Autodesk Inventor part; units mm, degrees
ref_plane "YZ Plane" through (0, 0, 0) normal (1, 0, 0) x (0, 1, 0)
ref_plane "XZ Plane" through (0, 0, 0) normal (0, 1, 0) x (-1, 0, 0)
ref_plane "XY Plane" through (0, 0, 0) normal (0, 0, 1) x (1, 0, 0)
sketch "Sketch1" plane through (0, 0, 0) normal (0, 0, 1) x (1, 0, 0)
  line L0 (7.62, 0) -> (72.898, 0)
  line L1 (80.518, 7.62) -> (80.518, 31.242)
  line L2 (72.898, 38.862) -> (7.62, 38.862)
  line L3 (0, 31.242) -> (0, 7.62)
  arc A0 (7.62, 38.862) -> (0, 31.242) centre (7.62, 31.242) ccw
  arc A1 (80.518, 31.242) -> (72.898, 38.862) centre (72.898, 31.242) ccw
  arc A2 (72.898, 0) -> (80.518, 7.62) centre (72.898, 7.62) ccw
  arc A3 (0, 7.62) -> (7.62, 0) centre (7.62, 7.62) ccw
  point P0 (0, 0)
  point P1 (80.518, 38.862)
  point P2 (80.518, 0)
  point P3 (0, 38.862)
  dimension "d0" = 80.518
  dimension "d1" = 38.862
  dimension "d2" = 7.62
  dimension "d3" = 7.62
  dimension "d4" = 7.62
  dimension "d5" = 7.62
extrude "Extrusion1" add sketch "Sketch1" along normal blind 80.518
sketch "Sketch2" plane through (7.62, 38.862, 0) normal (0, 1, 0) x (1, 0, 0)
  line L0 (14.986, -19.304) -> (55.118, -19.304)
  line L1 (60.198, -24.384) -> (60.198, -54.61)
  line L2 (55.118, -59.69) -> (14.986, -59.69)
  line L3 (9.906, -54.61) -> (9.906, -24.384)
  line L4 (65.278, -80.518) -> (0, -80.518)
  line L5 (72.898, 0) -> (72.898, -80.518)
  arc A0 (14.986, -19.304) -> (9.906, -24.384) centre (14.986, -24.384) ccw
  arc A1 (60.198, -24.384) -> (55.118, -19.304) centre (55.118, -24.384) ccw
  arc A2 (55.118, -59.69) -> (60.198, -54.61) centre (55.118, -54.61) ccw
  arc A3 (9.906, -54.61) -> (14.986, -59.69) centre (14.986, -54.61) ccw
  point P0 (-7.62, 0)
  point P1 (9.906, -19.304)
  point P2 (60.198, -19.304)
  point P3 (9.906, -59.69)
  dimension "d16" = 40.386
  dimension "d17" = 50.292
  dimension "d18" = 20.828
  dimension "d19" = 12.7
  dimension "d20" = 5.08
  dimension "d21" = 5.08
  dimension "d22" = 5.08
  dimension "d23" = 5.08
extrude "Extrusion2" cut sketch "Sketch2" against normal blind 27.178
sketch "Sketch3" plane through (0, 0, 80.518) normal (0, 0, 1) x (1, 0, 0)
  line L0 (14.732, 31.242) -> (65.532, 31.242)
  line L1 (70.612, 26.162) -> (70.612, 12.7)
  line L2 (65.532, 7.62) -> (14.732, 7.62)
  line L3 (9.652, 12.7) -> (9.652, 26.162)
  line L4 (80.518, 7.62) -> (80.518, 31.242)
  line L5 (72.898, 38.862) -> (7.62, 38.862)
  arc A0 (70.612, 26.162) -> (65.532, 31.242) centre (65.532, 26.162) ccw
  arc A1 (65.532, 7.62) -> (70.612, 12.7) centre (65.532, 12.7) ccw
  arc A2 (9.652, 12.7) -> (14.732, 7.62) centre (14.732, 12.7) ccw
  arc A3 (14.732, 31.242) -> (9.652, 26.162) centre (14.732, 26.162) ccw
  point P0 (0, 0)
  point P1 (9.652, 31.242)
  point P2 (70.612, 31.242)
  point P3 (9.652, 7.62)
  dimension "d26" = 60.96
  dimension "d27" = 9.906
  dimension "d28" = 23.622
  dimension "d29" = 7.62
  dimension "d30" = 5.08
  dimension "d31" = 5.08
extrude "Extrusion3" cut sketch "Sketch3" against normal blind 14.478
sketch "Sketch4" plane through (0, 0, 0) normal (0, 0, -1) x (-1, 0, 0)
  line L0 (-67.056, 32.004) -> (-13.716, 32.004)
  line L1 (-8.636, 26.924) -> (-8.636, 11.684)
  line L2 (-13.716, 6.604) -> (-67.056, 6.604)
  line L3 (-72.136, 11.684) -> (-72.136, 26.924)
  line L4 (0, 7.62) -> (0, 31.242)
  line L5 (-7.62, 38.862) -> (-72.898, 38.862)
  arc A0 (-67.056, 32.004) -> (-72.136, 26.924) centre (-67.056, 26.924) ccw
  arc A1 (-8.636, 26.924) -> (-13.716, 32.004) centre (-13.716, 26.924) ccw
  arc A2 (-13.716, 6.604) -> (-8.636, 11.684) centre (-13.716, 11.684) ccw
  arc A3 (-72.136, 11.684) -> (-67.056, 6.604) centre (-67.056, 11.684) ccw
  point P0 (0, 0)
  point P1 (-72.136, 32.004)
  point P2 (-8.636, 6.604)
  point P3 (-8.636, 32.004)
  dimension "d34" = 63.5
  dimension "d35" = 25.4
  dimension "d36" = 8.636
  dimension "d37" = 6.858
  dimension "d38" = 5.08
extrude "Extrusion4" cut sketch "Sketch4" against normal blind 14.478
The listing builds one solid part. Answer for the finished solid, in the listing's coordinates (mm). A direction names the side the tool comes from. Give positions to 0.01 mm unless a question says otherwise; leave off trailing zeros. Order: outer loops, then holes, each group sorted by start corner. A loop starts at its lowest first (then second) coordinate and runs counter-clockwise, first axis right, second up. Notation, with made-up numbers: (16.5, 39) - (57.5, 39) arc R22 ccw to (57.5, 70) - close; hole circle Ø9 at (-6, 13). An arc over 180 degrees is marked (long way). Answer as CSV lines item,"result".
Q1. Each of these flat-tipped pins is pushed along its axis until it touches: pin 1 Ø12 at (x, y) = (17.5, 19) entering from -Z; pin 2 Ø1 at (x, y) = (34, 15) entering from +Z. Where does it stop, or does it pass through?
Answer key:
pin 1,"stops at z = 14.48"
pin 2,"stops at z = 66.04"
Q2. A cutting plane is placed at A-A, the plane y = 21. Determine the outline of the cut face in (x, z), and give its area (3 significant figures).
Answer key:
outline,"(0, 0) - (8.64, 0) - (8.64, 14.48) - (72.14, 14.48) - (72.14, 0) - (80.52, 0) - (80.52, 80.52) - (70.61, 80.52) - (70.61, 66.04) - (9.65, 66.04) - (9.65, 80.52) - (0, 80.52) - close; hole (17.53, 24.38) arc R5.08 ccw to (22.61, 19.3) - (62.74, 19.3) arc R5.08 ccw to (67.82, 24.38) - (67.82, 54.61) arc R5.08 ccw to (62.74, 59.69) - (22.61, 59.69) arc R5.08 ccw to (17.53, 54.61) - close"
area,"2,670 mm^2"
Q3. Which of the six approach directions +Z, -Z, +X, -X, +Y, -Y give full straight-line access (tool end or side, diameter ignored) to faces 4 (the face through (40, 33, 80.518)), 5 (the face through (41, 32.004, 7)), 6 (the face through (43, 25, 59.69)), 7 (the face through (40, 7.62, 73))?
Answer key:
face 4,"+Z, +X, -X, +Y, -Y"
face 5,"-Z"
face 6,"+Y"
face 7,"+Z"
Q4. Determine the mould class of faces 1 (the face through (2.291, 2.173, 39.695)), 2 (the face through (40, 33, 0)), 3 (the face through (10.164, 8.053, 7.138)) for opening direction X: pulls with the +X half, pulls with the -X half, needs draft (parallel to the pull), parting line crosses it, or undercut.
Answer key:
face 1,"pulls with the -X half"
face 2,"needs draft"
face 3,"undercut"
Q5. A cutting plane is placed at C-C, the plane z = 36.5. Determine the outline of the cut face in (x, y).
Answer key:
outline,"(0, 7.62) arc R7.62 ccw to (7.62, 0) - (72.9, 0) arc R7.62 ccw to (80.52, 7.62) - (80.52, 31.24) arc R7.62 ccw to (72.9, 38.86) - (67.82, 38.86) - (67.82, 11.68) - (17.53, 11.68) - (17.53, 38.86) - (7.62, 38.86) arc R7.62 ccw to (0, 31.24) - close"
Q6. A cutting plane is placed at D-D, the plane x = 19. Determine the outline of the cut face in (y, z), and give its area (3 significant figures).
Answer key:
outline,"(0, 0) - (6.6, 0) - (6.6, 14.48) - (32, 14.48) - (32, 0) - (38.86, 0) - (38.86, 20.81) - (11.68, 20.81) - (11.68, 58.19) - (38.86, 58.19) - (38.86, 80.52) - (31.24, 80.52) - (31.24, 66.04) - (7.62, 66.04) - (7.62, 80.52) - (0, 80.52) - close"
area,"1,400 mm^2"
Q7. A cutting plane is placed at B-B, the plane z = 73.5. Determine the outline of the cut face in (x, y).
Answer key:
outline,"(0, 7.62) arc R7.62 ccw to (7.62, 0) - (72.9, 0) arc R7.62 ccw to (80.52, 7.62) - (80.52, 31.24) arc R7.62 ccw to (72.9, 38.86) - (7.62, 38.86) arc R7.62 ccw to (0, 31.24) - close; hole (9.65, 12.7) arc R5.08 ccw to (14.73, 7.62) - (65.53, 7.62) arc R5.08 ccw to (70.61, 12.7) - (70.61, 26.16) arc R5.08 ccw to (65.53, 31.24) - (14.73, 31.24) arc R5.08 ccw to (9.65, 26.16) - close"
Q8. Straight lines are drawn through the part: L1, parallel to Z at x = 24, y = 12; L2, parallel to X at y = 18.5, z = 76.5; L3, parallel to X at y = 15.5, z = 36. For each, find the intervals that lie inside material, in ascending order.
Answer key:
L1,"z = 14.48 to 19.3, 59.69 to 66.04"
L2,"x = 0 to 9.65, 70.61 to 80.52"
L3,"x = 0 to 17.53, 67.82 to 80.52"
